```python
from build123d import *

# Parameters (mm, degrees)
F0_W           = 100
F0_H           = 50
F1_DEPTH       = 5
F2_R           = 10
F3_DEPTH       = 10
F4_R           = 5.1
F5_DEPTH       = 25
F6_R           = 5
F7_R           = 2.65
F8_DEPTH       = 25
F11_R          = 2.6
F12_DEPTH      = 25
F12_DEPTH_BACK = 25


with BuildPart() as f1:
    # F0 (on Top) → F1 (new body)
    with BuildSketch(Plane.XY):
        Rectangle(F0_W, F0_H)
    extrude(amount=F1_DEPTH)

    # F2 (on face) → F3 (join)
    with BuildSketch(Plane.XY.offset(5)):
        Circle(F2_R)
    extrude(amount=F3_DEPTH)

    # F4 (on face) → F5 (cut)
    with BuildSketch(Plane.XY.offset(15)):
        Circle(F4_R)
    extrude(amount=-F5_DEPTH, mode=Mode.SUBTRACT)

    # F6
    f6_edges = [f1.edges().sort_by_distance(p)[0] for p in [
        (-50, -25, 2.5),
        (-50, 25, 2.5),
        (50, 25, 2.5),
        (50, -25, 2.5),
    ]]
    fillet(f6_edges, radius=F6_R)

    # F7 (on face) → F8 (cut)
    with BuildSketch(Plane.XY.offset(5)):
        with Locations((42.5, 17.5)):
            Circle(F7_R)
        with Locations((42.5, -17.5)):
            Circle(F7_R)
        with Locations((-42.5, -17.5)):
            Circle(F7_R)
        with Locations((-42.5, 17.5)):
            Circle(F7_R)
    extrude(amount=-F8_DEPTH, mode=Mode.SUBTRACT)

    # F9 (on Front) → F10 (revolve)
    with BuildSketch(Plane.XZ):
        Polygon((22.2268737853, 5.2352962084), (10.0123630837, 13.9599470422), (9.8070763052, 5.2352962084), align=None)
    revolve(axis=Axis((0, 0, 5), (0, 0, -1)))

    # F11 (on Right) → F12 (cut, two sides)
    with BuildSketch(Plane.YZ) as f12_sk:
        with Locations((0, 9.5)):
            Circle(F11_R)
    extrude(amount=-F12_DEPTH, mode=Mode.SUBTRACT)
    extrude(f12_sk.sketch, amount=F12_DEPTH_BACK, mode=Mode.SUBTRACT)


solid = f1.part
```
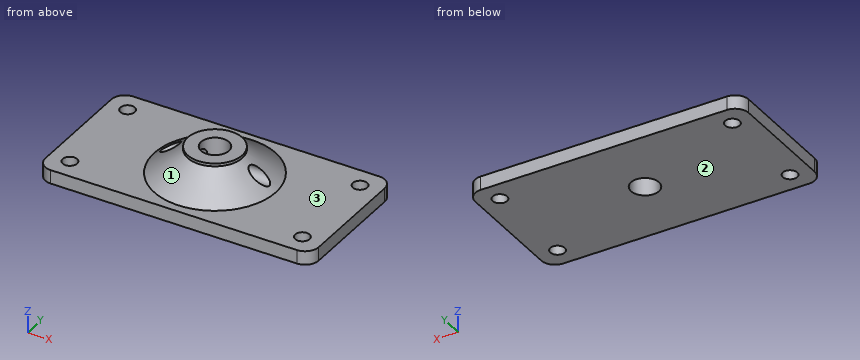
Check sheet for the modelled part. Datum: model origin and axes. Units: mm. Face numbers are marked on the shaded views. Give positions to 0.01 mm unless a question says otherwise; leave off trailing zeros. Write each loop counter-clockwise with the first axis right and the second up, starting at its lowest first coordinate (ties: lowest second). Pieces come first, ordered by that corner, then holes.
Item 1: Cross-section at C-C (x = 42.5). Enter the section's corners in (y, z).
Item 2: Gauge pin test, flat ends, axial feed: pin 1 (8 mm diameter, centred on x = 0, y = 0, fed in from +Z); pin 2 (7 mm diameter, centred on x = -42.5, y = 17.5, fed in from +Z). Record the tip position at first contact, or that the pin passes through.
Item 3: Scan lines: L1, parallel to Y at x = -42.5, z = 2.7; L2, parallel to Y at x = -44.5, z = 2.5; L3, parallel to Z at x = -45, y = -1.5. Record each from-to range of solid material in increasing order.
Item 4: Cross-section at D-D (y = 0). Enter the section's corners in (x, z).
Item 5: Cross-section at A-A (z = 2.75). Enter the section's corners in (x, y).
Item 6: Draft check along Z on the marked faces 1, 2 and 3. Enter one of: released by +Z, released by -Z, zero draft, split by the parting line, or undercut.
Item 7: Cross-section at B-B (x = 0). Enter the section's corners in (y, z).
Report:
1. outline: (-25, 0) - (-20.15, 0) - (-20.15, 5) - (-25, 5) - close; (-14.85, 0) - (14.85, 0) - (14.85, 5) - (-14.85, 5) - close; (20.15, 0) - (25, 0) - (25, 5) - (20.15, 5) - close
2. pin 1: passes through
2. pin 2: stops at z = 5
3. L1: y = -25 to -20.15, -14.85 to 14.85, 20.15 to 25
3. L2: y = -25 to -19.24, -15.76 to 15.76, 19.24 to 25
3. L3: z = 0 to 5
4. outline: (-50, 0) - (-5.1, 0) - (-5.1, 6.9) - (-19.9, 6.9) - (-22.23, 5.24) - (-10, 5.24) - (-10, 5) - (-50, 5) - close; (-12.62, 12.1) - (-5.1, 12.1) - (-5.1, 15) - (-10, 15) - (-10, 13.43) - (-10.01, 13.96) - close; (5.1, 0) - (50, 0) - (50, 5) - (10, 5) - (10, 5.24) - (22.23, 5.24) - (19.9, 6.9) - (5.1, 6.9) - close; (5.1, 12.1) - (12.62, 12.1) - (10.01, 13.96) - (10, 13.43) - (10, 15) - (5.1, 15) - close
5. outline: (-50, -20) arc R5 ccw to (-45, -25) - (45, -25) arc R5 ccw to (50, -20) - (50, 20) arc R5 ccw to (45, 25) - (-45, 25) arc R5 ccw to (-50, 20) - close; hole circle Ø5.3 at (-42.5, -17.5); hole circle Ø5.3 at (-42.5, 17.5); hole circle Ø10.2 at (0, 0); hole circle Ø5.3 at (42.5, -17.5); hole circle Ø5.3 at (42.5, 17.5)
6. face 1: released by +Z
6. face 2: released by -Z
6. face 3: undercut
7. outline: (-25, 0) - (-5.1, 0) - (-5.1, 15) - (-10, 15) - (-10, 13.43) - (-10.01, 13.96) - (-22.23, 5.24) - (-10, 5.24) - (-10, 5) - (-25, 5) - close; (5.1, 0) - (25, 0) - (25, 5) - (10, 5) - (10, 5.24) - (22.23, 5.24) - (10.01, 13.96) - (10, 13.43) - (10, 15) - (5.1, 15) - close
